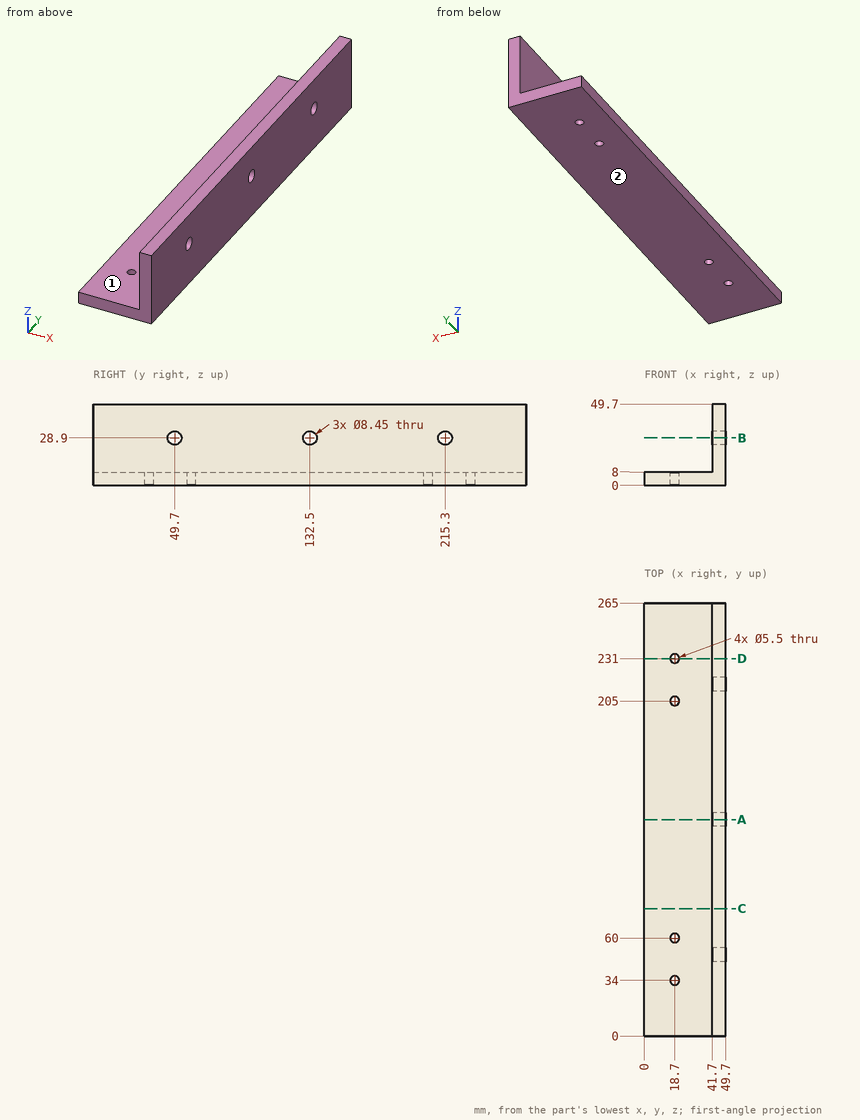
Here's the drawing with two shaded views (mm, measured from the low corner). I have some questions. A direction names the side the tool comes from. Coordinates: 2 decimals unless noted, no trailing zeros. Order: outer loops, then holes, each group sorted by start corner. A loop starts at its lowest first (then second) coordinate and runs counter-clockwise, first axis right, second up. Notation, with made-up numbers: (9, -35) -> (43, -35) arc R31 cw to (43, -10) -> close; hole circle Ø4 at (-19, 67). An arc over 180 degrees is marked (long way). Write each question's results on one line, items separated by ' | '.
Item 1: I want a section at A-A, the plane y = 132.5. Write out the boundary of the cut face in (x, z) (3 decimals), then the cut area to 3 significant figures.
Results are:
outline: (0, 0) -> (49.7, 0) -> (49.7, 24.675) -> (41.7, 24.675) -> (41.7, 8) -> (0, 8) -> close; (41.7, 33.125) -> (49.7, 33.125) -> (49.7, 49.7) -> (41.7, 49.7) -> close | area: 664 mm²
Item 2: Which directions (+Z, -Z, +X, -X, +Y, -Y) give clear straight access to the entire face, cutting with the end or side of a thin tool? Please do the marked faces 1 and 2.
Results are:
face 1: +Z, -X, +Y, -Y | face 2: -Z, +X, -X, +Y, -Y
Item 3: I want a section at B-B, the plane z = 28.9. Write out the boundary of the cut face in (x, y) (3 decimals), then the cut area to 3 significant figures.
Results are:
outline: (41.7, 0) -> (49.7, 0) -> (49.7, 45.475) -> (41.7, 45.475) -> close; (41.7, 53.925) -> (49.7, 53.925) -> (49.7, 128.275) -> (41.7, 128.275) -> close; (41.7, 136.725) -> (49.7, 136.725) -> (49.7, 211.075) -> (41.7, 211.075) -> close; (41.7, 219.525) -> (49.7, 219.525) -> (49.7, 265) -> (41.7, 265) -> close | area: 1,920 mm²
Item 4: I want a section at D-D, the plane y = 231. Write out the boundary of the cut face in (x, z), then the cut area to 3 significant figures.
Results are:
outline: (0, 0) -> (15.95, 0) -> (15.95, 8) -> (0, 8) -> close; (21.45, 0) -> (49.7, 0) -> (49.7, 49.7) -> (41.7, 49.7) -> (41.7, 8) -> (21.45, 8) -> close | area: 687 mm²
Item 5: I want a section at C-C, the plane y = 78. Write out the boundary of the cut face in (x, z), then the cut area to 3 significant figures.
Results are:
outline: (0, 0) -> (49.7, 0) -> (49.7, 49.7) -> (41.7, 49.7) -> (41.7, 8) -> (0, 8) -> close | area: 731 mm²
Item 6: If I drill on line 1 along Y through (x, z) = (45, 28.9) (3 decimals); line 2 along Z through (x, y) = (46.25, 215.3) (3 decimals); line 3 along X through (y, z) = (34, 2.5), over which ranges is the centre line in solid material (lowest first)?
Results are:
line 1: 0 to 45.475, 53.925 to 128.275, 136.725 to 211.075, 219.525 to 265 | line 2: 0 to 24.675, 33.125 to 49.7 | line 3: 0 to 15.95, 21.45 to 49.7
Item 7: I'm going to push flat-ended pins straight in: pin 1 Ø21 at (y, z) = (100.5, 30) entering from -X; pin 2 Ø12 at (y, z) = (130.5, 28.5) entering from +X; pin 3 Ø9 at (x, y) = (18.7, 205) entering from +Z. Where does each tip first touch, or does it pass through?
Results are:
pin 1: x = 41.7 | pin 2: x = 49.7 | pin 3: z = 8
